Can you work these out from the model? Positions are in its coordinate system, mm. Face numbers are marked on the shaded views. A direction names the side the tool comes from. Round coordinates to 2 decimals unless told otherwise and drop trailing zeros. Order: outer loops, then holes, each group sorted by start corner. A loop starts at its lowest first (then second) coordinate and runs counter-clockwise, first axis right, second up. Notation, with made-up numbers: M 60.5,-7 L 96.5,-7 A19 ccw 96.5,2 Z; hole C 49,4 d11. An arc over 180 degrees is marked long. One line per question, with ' | ' between items.
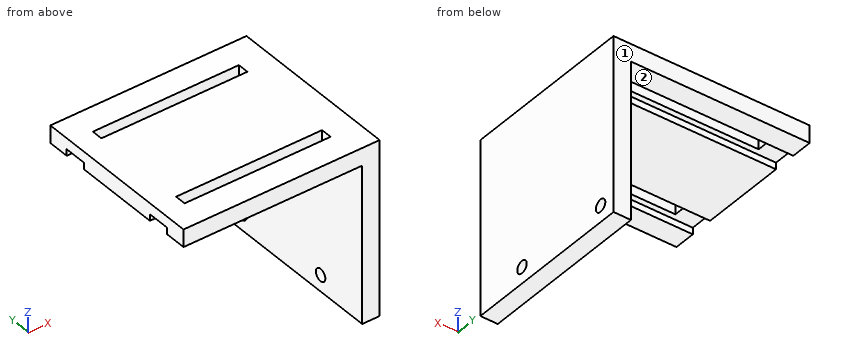
```python
from build123d import *

# Parameters (mm, degrees)
F1_DEPTH = 50.8
F2_R     = 1.8
F3_DEPTH = 25.4
F4_W     = 42.545
F4_H     = 3.2512
F5_DEPTH = 25.4
F6_W     = 52.07
F6_H     = 6.604
F7_DEPTH = 1.905


with BuildPart() as f1:
    # F0 (on Front) → F1 (new body)
    with BuildSketch(Plane.XZ):
        Polygon((-5.08, 0), (0, 0), (0, 50.8), (-57.15, 50.8), (-57.15, 45.72), (-5.08, 45.72), align=None)
    extrude(amount=F1_DEPTH)

    # F2 (on face) → F3 (cut)
    with BuildSketch(Plane.YZ):
        with Locations((-34.925, 4.7625)):
            Circle(F2_R)
        with Locations((-4.925, 4.7625)):
            Circle(F2_R)
    extrude(amount=-F3_DEPTH, mode=Mode.SUBTRACT)

    # F4 (on face) → F5 (cut)
    with BuildSketch(Plane.XY.offset(50.8)):
        with Locations((-29.5275, -41.275)):
            Rectangle(F4_W, F4_H)
        with Locations((-29.5275, -9.525)):
            Rectangle(F4_W, F4_H)
    extrude(amount=-F5_DEPTH, mode=Mode.SUBTRACT)

    # F6 (on face) → F7 (cut)
    with BuildSketch(Plane(origin=(0, 0, 45.72), x_dir=(1, 0, 0), z_dir=(0, 0, -1))):
        with Locations((-31.115, 41.275)):
            Rectangle(F6_W, F6_H)
        with Locations((-31.115, 9.525)):
            Rectangle(F6_W, F6_H)
    extrude(amount=-F7_DEPTH, mode=Mode.SUBTRACT)


solid = f1.part
```
(1) Please list where these lines run through material, in increasing order: probe 1 along Y at (x, z) = (-13, 48.5); probe 2 along X at (y, z) = (-8.5, 46); probe 3 along Z at (x, y) = (-14, -3). Write a range as [from, to].
Final values:
probe 1: [-50.8, -42.9], [-39.65, -11.15], [-7.9, 0] | probe 2: [-5.08, 0] | probe 3: [45.72, 50.8]
(2) If we section it at A-A on x = -32: Please give me the cut outline in (y, z) (3 decimals), plus the area to 3 significant figures.
Final values:
outline: M -50.8,45.72 L -44.577,45.72 L -44.577,47.625 L -42.901,47.625 L -42.901,50.8 L -50.8,50.8 Z; M -39.649,47.625 L -37.973,47.625 L -37.973,45.72 L -12.827,45.72 L -12.827,47.625 L -11.151,47.625 L -11.151,50.8 L -39.649,50.8 Z; M -7.899,47.625 L -6.223,47.625 L -6.223,45.72 L 0,45.72 L 0,50.8 L -7.899,50.8 Z | area: 212 mm^2
(3) If we section it at B-B on y = -9.5: Please give me the cut outline in (x, z) (3 decimals).
Final values:
outline: M -57.15,47.625 L -50.8,47.625 L -50.8,50.8 L -57.15,50.8 Z; M -8.255,47.625 L -5.08,47.625 L -5.08,0 L 0,0 L 0,50.8 L -8.255,50.8 Z
(4) If we section it at D-D on y = -24: Please give me the cut outline in (x, z), plus the area to 3 significant figures.
Final values:
outline: M -57.15,45.72 L -5.08,45.72 L -5.08,0 L 0,0 L 0,50.8 L -57.15,50.8 Z | area: 523 mm^2
(5) On a 3-axis mill with a long thin cutter (end or side, diameter ignored), from which of +Z, -Z, +X, -X, +Y, -Y can I reach the whole of each face in a straight line? I mean the marked faces 1 and 2. Say none if no direction works.
Final values:
face 1: +Z, -Z, +X, -X, +Y | face 2: -Z, -X, +Y, -Y
(6) Will these pins go through, and if not, where does the flat tip stop? pin 1 Ø2 at (x, y) = (-18.5, -5.5) entering from -Z; pin 2 Ø3.5 at (x, y) = (-39, -10) entering from -Z (3 decimals).
Final values:
pin 1: z = 45.72 | pin 2: z = 47.625
(7) If we section it at C-C on x = -7: Please give me the cut outline in (y, z) (3 decimals), plus the area to 3 significant figures.
Final values:
outline: M -50.8,45.72 L -44.577,45.72 L -44.577,47.625 L -37.973,47.625 L -37.973,45.72 L -12.827,45.72 L -12.827,47.625 L -6.223,47.625 L -6.223,45.72 L 0,45.72 L 0,50.8 L -50.8,50.8 Z | area: 233 mm^2
